CAD build for the part. Positions are in the model's coordinates, mm. Face numbers are marked on the shaded views. Coordinates: 2 decimals unless noted, no trailing zeros. Loops run counter-clockwise (first coordinate to the right, second up) from the corner with the lowest first, then second, coordinate; pieces in that order, holes last. Notation, with made-up numbers: (2, 83) -> (35, 83) arc R31 ccw to (35, 121) -> close; hole circle Ø11 at (50, 29). An arc over 180 degrees is marked (long way). Write each question's results on one line, items separated by ' | '.
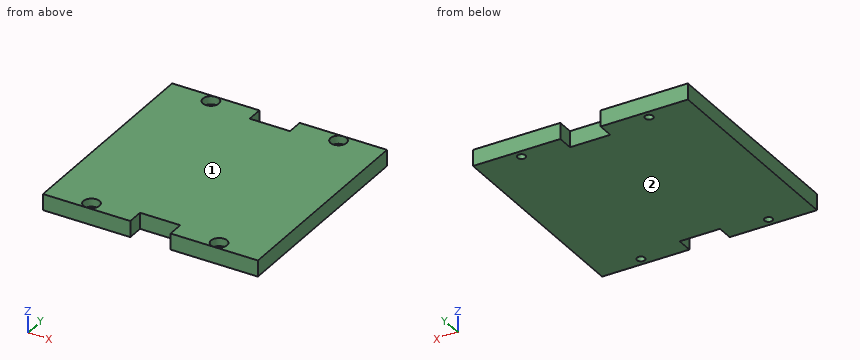
from build123d import *

# Parameters (mm, degrees)
ESQUISSE1_W             = 80
ESQUISSE1_H             = 80
BOSS_EXTRU_1_DEPTH      = 6
ESQUISSE2_R             = 1.5
ESQUISSE2_W             = 15
ESQUISSE2_H             = 6
ENL_V_MAT_EXTRU_1_DEPTH = 6
ESQUISSE3_R             = 2.995
ENL_V_MAT_EXTRU_2_DEPTH = 3


with BuildPart() as part:
    # Esquisse1 → Boss.-Extru.1 (new body)
    with BuildSketch(Plane.XY):
        with Locations((-40, 40)):
            Rectangle(ESQUISSE1_W, ESQUISSE1_H)
    extrude(amount=BOSS_EXTRU_1_DEPTH)

    # Esquisse2 → Enlèv. mat.-Extru.1 (cut)
    with BuildSketch(Plane.XY.offset(6)):
        with Locations((-16.25, 3)):
            Circle(ESQUISSE2_R)
        with Locations(Location((-63.75, 77, 0), (0, 0, 180))):
            Circle(ESQUISSE2_R)
        with Locations(Location((-16.25, 77, 0), (0, 0, 180))):
            Circle(ESQUISSE2_R)
        with Locations((-63.75, 3)):
            Circle(ESQUISSE2_R)
        with Locations((-40, 3)):
            Rectangle(ESQUISSE2_W, ESQUISSE2_H)
        with Locations((-40, 77)):
            Rectangle(ESQUISSE2_W, ESQUISSE2_H)
    extrude(amount=-ENL_V_MAT_EXTRU_1_DEPTH, mode=Mode.SUBTRACT)

    # Esquisse3 → Enlèv. mat.-Extru.2 (cut)
    with BuildSketch(Plane.XY.offset(6)):
        with Locations((-16.25, 3)):
            Circle(ESQUISSE3_R)
        with Locations((-63.75, 3)):
            Circle(ESQUISSE3_R)
        with Locations((-16.25, 77)):
            Circle(ESQUISSE3_R)
        with Locations((-63.75, 77)):
            Circle(ESQUISSE3_R)
    extrude(amount=-ENL_V_MAT_EXTRU_2_DEPTH, mode=Mode.SUBTRACT)


solid = part.part
1) Pin check, flat tips, straight feed: pin 1 (1 mm diameter, centred on x = -23.5, y = 66.5, fed in from -Z); pin 2 (3 mm diameter, centred on x = -37.5, z = 2, fed in from -Y); pin 3 (1.8 mm diameter, centred on x = -17, y = 2.5, fed in from +Z). Stop position of each tip, or through.
Outcome:
pin 1: stops at z = 0 | pin 2: stops at y = 6 | pin 3: stops at z = 3
2) Drill centre lines: L1, parallel to Y at x = -63.75, z = 0.7; L2, parallel to X at y = 3.5, z = 3.8. Where is each one in solid material? Low to high. Write a range as from..to.
Outcome:
L1: y = 0..1.5, 4.5..75.5, 78.5..80 | L2: x = -80..-66.7, -60.8..-47.5, -32.5..-19.2, -13.3..0
3) Slice it at A-A (x = -16.25). Write the cut outline in (y, z) (3 decimals).
Outcome:
outline: (0, 0) -> (1.5, 0) -> (1.5, 3) -> (0.005, 3) -> (0.005, 6) -> (0, 6) -> close; (4.5, 0) -> (75.5, 0) -> (75.5, 3) -> (74.005, 3) -> (74.005, 6) -> (5.995, 6) -> (5.995, 3) -> (4.5, 3) -> close; (78.5, 0) -> (80, 0) -> (80, 6) -> (79.995, 6) -> (79.995, 3) -> (78.5, 3) -> close
4) Two-plate mould, pull along Z, no slides. Class the marked faces 1 and 2: pulls with the +Z half, pulls with the -Z half, needs draft (parallel to the pull), parting line crosses it, or undercut.
Outcome:
face 1: pulls with the +Z half | face 2: pulls with the -Z half
5) Slice it at C-C (z = 4.75). Write the cut outline in (x, y) (3 decimals).
Outcome:
outline: (-80, 0) -> (-47.5, 0) -> (-47.5, 6) -> (-32.5, 6) -> (-32.5, 0) -> (0, 0) -> (0, 80) -> (-32.5, 80) -> (-32.5, 74) -> (-47.5, 74) -> (-47.5, 80) -> (-80, 80) -> close; hole circle Ø5.99 at (-63.75, 3); hole circle Ø5.99 at (-63.75, 77); hole circle Ø5.99 at (-16.25, 3); hole circle Ø5.99 at (-16.25, 77)
6) Slice it at B-B (y = 77). Write the cut outline in (x, z) (3 decimals).
Outcome:
outline: (-80, 0) -> (-65.25, 0) -> (-65.25, 3) -> (-66.745, 3) -> (-66.745, 6) -> (-80, 6) -> close; (-62.25, 0) -> (-47.5, 0) -> (-47.5, 6) -> (-60.755, 6) -> (-60.755, 3) -> (-62.25, 3) -> close; (-32.5, 0) -> (-17.75, 0) -> (-17.75, 3) -> (-19.245, 3) -> (-19.245, 6) -> (-32.5, 6) -> close; (-14.75, 0) -> (0, 0) -> (0, 6) -> (-13.255, 6) -> (-13.255, 3) -> (-14.75, 3) -> close
